```python
from build123d import *

# Parameters (mm, degrees)
SKETCH2_R               = 50.8
SKETCH2_R_2             = 41.275
BASE_CYLINDER_DEPTH     = 292.1
SKETCH3_R               = 69.85
SKETCH3_R_2             = 41.275
AFT_FLANGE_DEPTH        = 17.78
SKETCH4_R               = 69.85
SKETCH4_R_2             = 41.275
FORWARD_FLANGE_DEPTH    = 17.78
SKETCH6_R               = 50.0761
SKETCH6_R_2             = 47.0027
O_RING_SLOT_1_DEPTH     = 1.9812
SKETCH7_R               = 50.0761
SKETCH7_R_2             = 47.0027
O_RING_SLOT_2_DEPTH     = 1.9812
SKETCH8_R               = 3.175
CUT_EXTRUDE4_DEPTH      = 1
CUT_EXTRUDE4_DEPTH_BACK = 293.1
FILLET1_R               = 4.7625
SKETCH9_R               = 3.175
CUT_EXTRUDE5_DEPTH      = 7.62
SKETCH10_R              = 3.175
CUT_EXTRUDE6_DEPTH      = 7.62
CUT_EXTRUDE7_REACH      = 286.48
SKETCH11_R              = 1.4097
CUT_EXTRUDE8_REACH      = 286.48
SKETCH12_R              = 1.4097


with BuildPart() as part:
    # Sketch2 → Base Cylinder (new body)
    with BuildSketch(Plane(origin=(0, 0, 0), x_dir=(1, 0, 0), z_dir=(0, 1, 0))):
        Circle(SKETCH2_R)
        Circle(SKETCH2_R_2, mode=Mode.SUBTRACT)
    extrude(amount=BASE_CYLINDER_DEPTH)

    # Sketch3 → Aft Flange (add)
    with BuildSketch(Plane.XZ):
        Circle(SKETCH3_R)
        Circle(SKETCH3_R_2, mode=Mode.SUBTRACT)
    extrude(amount=-AFT_FLANGE_DEPTH)

    # Sketch4 → Forward Flange (add)
    with BuildSketch(Plane(origin=(0, 292.1, 0), x_dir=(1, 0, 0), z_dir=(0, 1, 0))):
        Circle(SKETCH4_R)
        Circle(SKETCH4_R_2, mode=Mode.SUBTRACT)
    extrude(amount=-FORWARD_FLANGE_DEPTH)

    # Sketch6 → O-Ring Slot 1 (cut)
    with BuildSketch(Plane.XZ):
        Circle(SKETCH6_R)
        Circle(SKETCH6_R_2, mode=Mode.SUBTRACT)
    extrude(amount=-O_RING_SLOT_1_DEPTH, mode=Mode.SUBTRACT)

    # Sketch7 → O-Ring Slot 2 (cut)
    with BuildSketch(Plane(origin=(0, 292.1, 0), x_dir=(1, 0, 0), z_dir=(0, 1, 0))):
        Circle(SKETCH7_R)
        Circle(SKETCH7_R_2, mode=Mode.SUBTRACT)
    extrude(amount=-O_RING_SLOT_2_DEPTH, mode=Mode.SUBTRACT)

    # Sketch8 → Cut-Extrude4 (cut, two sides)
    with BuildSketch(Plane.XZ) as cut_extrude4_sk:
        with Locations((-59.9186, 0)):
            Circle(SKETCH8_R)
        with Locations((-42.368848379, 42.368848379)):
            Circle(SKETCH8_R)
        with Locations((0, 59.9186)):
            Circle(SKETCH8_R)
        with Locations((42.368848379, 42.368848379)):
            Circle(SKETCH8_R)
        with Locations((59.9186, 0)):
            Circle(SKETCH8_R)
        with Locations((42.368848379, -42.368848379)):
            Circle(SKETCH8_R)
        with Locations((0, -59.9186)):
            Circle(SKETCH8_R)
        with Locations((-42.368848379, -42.368848379)):
            Circle(SKETCH8_R)
    extrude(amount=CUT_EXTRUDE4_DEPTH, mode=Mode.SUBTRACT)
    extrude(cut_extrude4_sk.sketch, amount=-CUT_EXTRUDE4_DEPTH_BACK, mode=Mode.SUBTRACT)

    # Fillet1
    fillet1_edges = [part.edges().sort_by_distance(p)[0] for p in [
        (-50.8, 17.78, 0),
        (-50.8, 274.32, 0),
    ]]
    fillet(fillet1_edges, radius=FILLET1_R)

    # Sketch9 → Cut-Extrude5 (cut)
    with BuildSketch(Plane(origin=(0, 292.1, 0), x_dir=(1, 0, 0), z_dir=(0, 1, 0))):
        with Locations((-22.929855511, 55.357568157)):
            Circle(SKETCH9_R)
        with Locations((22.929855511, -55.357568157)):
            Circle(SKETCH9_R)
        with Locations((22.929855511, 55.357568157)):
            Circle(SKETCH9_R)
        with Locations((-22.929855511, -55.357568157)):
            Circle(SKETCH9_R)
    extrude(amount=-CUT_EXTRUDE5_DEPTH, mode=Mode.SUBTRACT)

    # Sketch10 → Cut-Extrude6 (cut)
    with BuildSketch(Plane.XZ):
        with Locations((-22.929855511, 55.357568157)):
            Circle(SKETCH10_R)
        with Locations((22.929855511, -55.357568157)):
            Circle(SKETCH10_R)
        with Locations((22.929855511, 55.357568157)):
            Circle(SKETCH10_R)
        with Locations((-22.929855511, -55.357568157)):
            Circle(SKETCH10_R)
    extrude(amount=-CUT_EXTRUDE6_DEPTH, mode=Mode.SUBTRACT)

    # Sketch11 → Cut-Extrude7 (cut, up to next)
    with BuildSketch(Plane(origin=(0, 284.48, 0), x_dir=(1, 0, 0), z_dir=(0, 1, 0)), mode=Mode.PRIVATE) as cut_extrude7_sk1:
        with Locations((-22.929855511, 55.357568157)):
            Circle(SKETCH11_R)
    cut_extrude7_tool1 = extrude(cut_extrude7_sk1.sketch, amount=-CUT_EXTRUDE7_REACH, mode=Mode.PRIVATE) & part.part
    add(cut_extrude7_tool1.solids().sort_by_distance((-22.929856, 284.48, -55.357568))[0], mode=Mode.SUBTRACT)
    # Sketch11 → Cut-Extrude7 (cut, up to next)
    with BuildSketch(Plane(origin=(0, 284.48, 0), x_dir=(1, 0, 0), z_dir=(0, 1, 0)), mode=Mode.PRIVATE) as cut_extrude7_sk2:
        with Locations((22.929855511, 55.357568157)):
            Circle(SKETCH11_R)
    cut_extrude7_tool2 = extrude(cut_extrude7_sk2.sketch, amount=-CUT_EXTRUDE7_REACH, mode=Mode.PRIVATE) & part.part
    add(cut_extrude7_tool2.solids().sort_by_distance((22.929856, 284.48, -55.357568))[0], mode=Mode.SUBTRACT)
    # Sketch11 → Cut-Extrude7 (cut, up to next)
    with BuildSketch(Plane(origin=(0, 284.48, 0), x_dir=(1, 0, 0), z_dir=(0, 1, 0)), mode=Mode.PRIVATE) as cut_extrude7_sk3:
        with Locations((-22.929855511, -55.357568157)):
            Circle(SKETCH11_R)
    cut_extrude7_tool3 = extrude(cut_extrude7_sk3.sketch, amount=-CUT_EXTRUDE7_REACH, mode=Mode.PRIVATE) & part.part
    add(cut_extrude7_tool3.solids().sort_by_distance((-22.929856, 284.48, 55.357568))[0], mode=Mode.SUBTRACT)
    # Sketch11 → Cut-Extrude7 (cut, up to next)
    with BuildSketch(Plane(origin=(0, 284.48, 0), x_dir=(1, 0, 0), z_dir=(0, 1, 0)), mode=Mode.PRIVATE) as cut_extrude7_sk4:
        with Locations((22.929855511, -55.357568157)):
            Circle(SKETCH11_R)
    cut_extrude7_tool4 = extrude(cut_extrude7_sk4.sketch, amount=-CUT_EXTRUDE7_REACH, mode=Mode.PRIVATE) & part.part
    add(cut_extrude7_tool4.solids().sort_by_distance((22.929856, 284.48, 55.357568))[0], mode=Mode.SUBTRACT)

    # Sketch12 → Cut-Extrude8 (cut, up to next)
    with BuildSketch(Plane.XZ.offset(-7.62), mode=Mode.PRIVATE) as cut_extrude8_sk1:
        with Locations((-22.929855511, 55.357568157)):
            Circle(SKETCH12_R)
    cut_extrude8_tool1 = extrude(cut_extrude8_sk1.sketch, amount=-CUT_EXTRUDE8_REACH, mode=Mode.PRIVATE) & part.part
    add(cut_extrude8_tool1.solids().sort_by_distance((-22.929856, 7.62, 55.357568))[0], mode=Mode.SUBTRACT)
    # Sketch12 → Cut-Extrude8 (cut, up to next)
    with BuildSketch(Plane.XZ.offset(-7.62), mode=Mode.PRIVATE) as cut_extrude8_sk2:
        with Locations((22.929855511, 55.357568157)):
            Circle(SKETCH12_R)
    cut_extrude8_tool2 = extrude(cut_extrude8_sk2.sketch, amount=-CUT_EXTRUDE8_REACH, mode=Mode.PRIVATE) & part.part
    add(cut_extrude8_tool2.solids().sort_by_distance((22.929856, 7.62, 55.357568))[0], mode=Mode.SUBTRACT)
    # Sketch12 → Cut-Extrude8 (cut, up to next)
    with BuildSketch(Plane.XZ.offset(-7.62), mode=Mode.PRIVATE) as cut_extrude8_sk3:
        with Locations((-22.929855511, -55.357568157)):
            Circle(SKETCH12_R)
    cut_extrude8_tool3 = extrude(cut_extrude8_sk3.sketch, amount=-CUT_EXTRUDE8_REACH, mode=Mode.PRIVATE) & part.part
    add(cut_extrude8_tool3.solids().sort_by_distance((-22.929856, 7.62, -55.357568))[0], mode=Mode.SUBTRACT)
    # Sketch12 → Cut-Extrude8 (cut, up to next)
    with BuildSketch(Plane.XZ.offset(-7.62), mode=Mode.PRIVATE) as cut_extrude8_sk4:
        with Locations((22.929855511, -55.357568157)):
            Circle(SKETCH12_R)
    cut_extrude8_tool4 = extrude(cut_extrude8_sk4.sketch, amount=-CUT_EXTRUDE8_REACH, mode=Mode.PRIVATE) & part.part
    add(cut_extrude8_tool4.solids().sort_by_distance((22.929856, 7.62, -55.357568))[0], mode=Mode.SUBTRACT)


solid = part.part
```
Can you work these out from the model? Positions are in its coordinate system, mm. A direction names the side the tool comes from. Round coordinates to 2 decimals unless told otherwise and drop trailing zeros. Loops run counter-clockwise (first coordinate to the right, second up) from the corner with the lowest first, then second, coordinate; pieces in that order, holes last. Notation, with made-up numbers: M 42.5,62 L 66.5,62 A14 ccw 66.5,84 Z; hole C -19.5,40 d5. An arc over 180 degrees is marked long. Write item = value, one per line. Start each with the question number.
(1) Which directions (+Z, -Z, +X, -X, +Y, -Y) give clear straight access to the entire face, cutting with the end or side of a thin tool? Please do faces 1 (the face through (-21.465, 288.343, -52.541)), 2 (the face through (46.2, 0, -20.4)), 3 (the face through (24.39, 3.76, 52.54)), 4 (the face through (-0.688, 8.766, -63.018)), 5 (the face through (-52, 17.78, 21)).
(2) I need wall thicknesses on line 1 along Y through (x, z) = (14, -55); line 2 along X through (y, z) = (237, 5.5); line 3 along X through (y, z) = (278.5, -14.5). Which ranges of each line are inside material? Lowest first, please.
(3) Suppose I cut it at C-C on y = 228. Write out the boundary of the cut face in (x, z) (3 decimals), plus the area to 3 significant figures.
(4) I'm going to push flat-ended pins straight in: P1, Ø2, axis at y = 175.5, z = 42.5, coming from the +X side; P2, Ø4, axis at x = 45.5, y = 218.5, coming from the +Z side; P3, Ø1.9, axis at x = 21.5, z = 56.5, coming from the -Y side; P4, Ø4, axis at x = 42.37, z = -42.37, coming from the +Y side. Where does each tip first touch, or does it pass through?
(5) If we mould it in two halves opening along X, with no side actions, what happens to faces 6 (the face through (62.95, 283.09, 0.95)), 7 (the face through (-55.431, 8.766, -42.503)), 8 (the face through (44.076, 283.086, 45.046)), 9 (the face through (0, 0, -42))? For each: released by +X, released by -X, zero draft, split by the parting line, or undercut.
(6) Suppose I cut it at A-A on z = 0. Give the number of separate pieces and of enclosed holes in the cut face, plus the area to 3 significant figures.
Answer block:
q1.face_1 = +Y
q1.face_2 = +Z, -Z, +X, -X, -Y
q1.face_3 = -Y
q1.face_4 = +Y, -Y
q1.face_5 = none
q2.line_1 = 0 to 17.78, 274.32 to 292.1
q2.line_2 = -50.5 to -40.91, 40.91 to 50.5
q2.line_3 = -68.33 to -38.64, 38.64 to 68.33
q3.outline = C 0,0 d101.6; hole C 0,0 d82.55
q3.area = 2,760 mm²
q4.P1 = 29.3
q4.P2 = 26.24
q4.P3 = 7.62
q4.P4 = through
q5.face_6 = undercut
q5.face_7 = split by the parting line
q5.face_8 = undercut
q5.face_9 = zero draft
q6.separate_pieces = 6
q6.enclosed_holes = 0
q6.area = 6,460 mm²
